Input: dimensioned drawing with shaded views. Units: mm. Origin: part minimum x, y, z. Coordinates: 2 decimals unless noted, no trailing zeros. Loops run counter-clockwise (first coordinate to the right, second up) from the corner with the lowest first, then second, coordinate; pieces in that order, holes last.
Item 1: Section query D-D, the plane y = 17.5. Return the cut outline in (x, z), then the cut area to 3 significant figures.
Item 2: Pin query (flat end, axial travel): pin 1 Ø3 at (x, y) = (12.5, 7.5) entering from -Z. Return the tip coordinate at first contact, or that it passes through.
Item 3: Line query: probe 1 along Y at (x, z) = (12.5, 1.1); probe 2 along Y at (x, z) = (106.28, 3.75); probe 3 along X at (y, z) = (16, 1). Output: solid intervals per line, ascending.
Item 4: Section query B-B, the plane y = 42.5. Return the cut outline in (x, z), then the cut area to 3 significant figures.
Item 5: Section query A-A, the plane x = 106.28. Return the cut outline in (y, z).
Item 6: Section query C-C, the plane y = 7.5. Return the cut outline in (x, z).
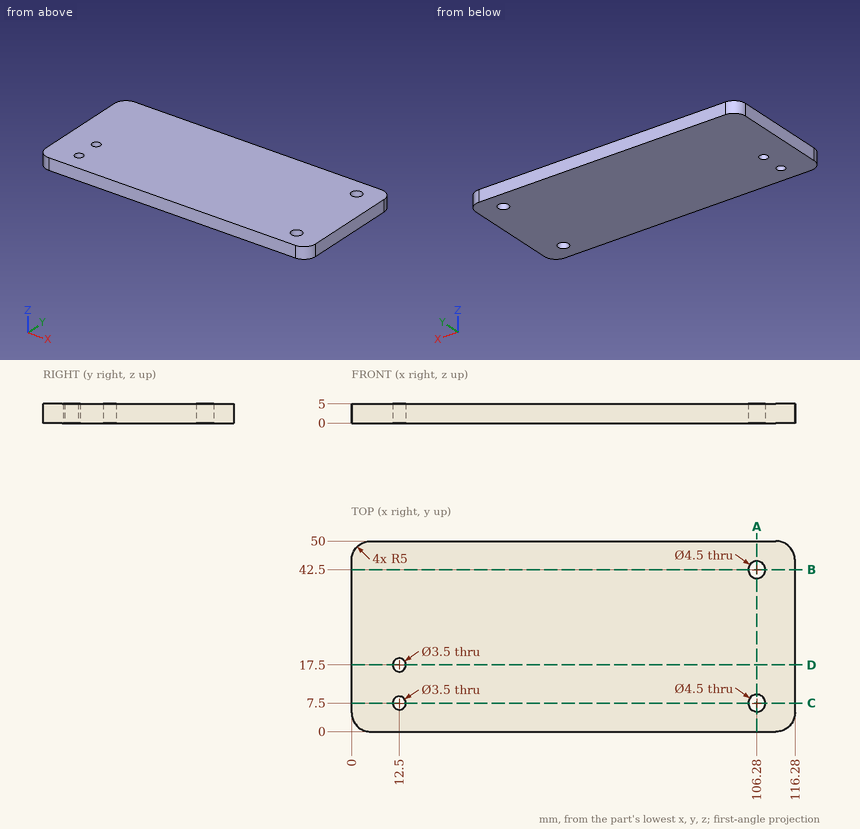
Verdict:
1. outline: (0, 0) - (10.75, 0) - (10.75, 5) - (0, 5) - close; (14.25, 0) - (116.28, 0) - (116.28, 5) - (14.25, 5) - close
1. area: 564 mm2
2. pin 1: passes through
3. probe 1: y = 0 to 5.75, 9.25 to 15.75, 19.25 to 50
3. probe 2: y = 0 to 5.25, 9.75 to 40.25, 44.75 to 50
3. probe 3: x = 0 to 11.6, 13.4 to 116.28
4. outline: (0, 0) - (104.03, 0) - (104.03, 5) - (0, 5) - close; (108.53, 0) - (116.28, 0) - (116.28, 5) - (108.53, 5) - close
4. area: 559 mm2
5. outline: (0, 0) - (5.25, 0) - (5.25, 5) - (0, 5) - close; (9.75, 0) - (40.25, 0) - (40.25, 5) - (9.75, 5) - close; (44.75, 0) - (50, 0) - (50, 5) - (44.75, 5) - close
6. outline: (0, 0) - (10.75, 0) - (10.75, 5) - (0, 5) - close; (14.25, 0) - (104.03, 0) - (104.03, 5) - (14.25, 5) - close; (108.53, 0) - (116.28, 0) - (116.28, 5) - (108.53, 5) - close
